CAD build for the part. Positions are in the model's coordinates, mm. A direction names the side the tool comes from. Round coordinates to 2 decimals unless told otherwise and drop trailing zeros. Loops run counter-clockwise (first coordinate to the right, second up) from the corner with the lowest first, then second, coordinate; pieces in that order, holes last. Notation, with made-up numbers: (-29.75, 38) - (-13.75, 38) arc R24 cw to (-13.75, 59) - close; hole circle Ø11 at (37.25, -28.75). An arc over 180 degrees is marked (long way). Use one line per item in the form item = value.
Solid Edge part; units mm, degrees
sketch "Sketch1" plane through (0, 0, 0) normal (0, -1, 0) x (1, 0, 0)
  line L0 (0, 0) -> (0, 40)
  line L1 (0, 40) -> (4, 40)
  line L2 (4, 40) -> (4, 4)
  line L3 (4, 4) -> (100, 4)
  line L4 (100, 4) -> (100, 0)
  line L5 (100, 0) -> (0, 0)
  dimension "D1" = 100
  dimension "D2" = 100
extrude "Protrusion1" add sketch "Sketch1" along normal mid plane 16
hole "Hole1" at (0, 0, 14) direction (1, 0, 0) diameter 2.459 end up to next
hole "Hole2" at (0, 0, 34) direction (1, 0, 0) diameter 2.459 end up to next
hole "Bohrung_3" at (14.002, 0, 0) direction (0, 0, 1) diameter 2.459 end up to next
hole "Hole3" at (90, 0, 0) direction (0, 0, 1) diameter 2.459 end up to next
properties material "Aluminiumlegierung:3.3535 , AlMg3, EN-AW 5754"
1) Two-plate mould, pull along Z, no slides. Class faces 1 (the flat face through (51, 0, 4)), 2 (the flat face through (100, 0, 2)), 3 (the cylindrical face through (1.972, 0.369, 15.173)): +Z half, -Z half, draft (parallel to the pull), parting line (faces both ways), or undercut.
Report:
face_1 = +Z half
face_2 = draft
face_3 = undercut
2) Slice it at A-A (x = 90). Write the cut outline in (y, z), plus the area to 3 significant figures.
Report:
outline = (-8, 0) - (-1.23, 0) - (-1.23, 4) - (-8, 4) - close; (1.23, 0) - (8, 0) - (8, 4) - (1.23, 4) - close
area = 54.2 mm^2
3) Slice it at D-D (x = 74.5). Write the cut outline in (y, z).
Report:
outline = (-8, 0) - (8, 0) - (8, 4) - (-8, 4) - close
4) Slice it at B-B (y = 0). Write the cut outline in (x, z), plus the area to 3 significant figures.
Report:
outline = (0, 0) - (12.77, 0) - (12.77, 4) - (4, 4) - (4, 12.77) - (0, 12.77) - close; (0, 15.23) - (4, 15.23) - (4, 32.77) - (0, 32.77) - close; (0, 35.23) - (4, 35.23) - (4, 40) - (0, 40) - close; (15.23, 0) - (88.77, 0) - (88.77, 4) - (15.23, 4) - close; (91.23, 0) - (100, 0) - (100, 4) - (91.23, 4) - close
area = 505 mm^2
5) Tool access for faces 4 (the cylindrical face through (1.97, 0.05, 32.77)), 5 (the flat face through (4, 0, 22)): list every direction of +Z, -Z, +X, -X, +Y, -Y with a clear straight run to the whole face (end or side of a thin tool).
Report:
face_4 = +X, -X
face_5 = +Z, +X, +Y, -Y
6) Slice it at C-C (z = 34). Write the cut outline in (x, y), plus the area to 3 significant figures.
Report:
outline = (0, -8) - (4, -8) - (4, -1.23) - (0, -1.23) - close; (0, 1.23) - (4, 1.23) - (4, 8) - (0, 8) - close
area = 54.2 mm^2
7) Drill centre lines: probe 1 along Z at (x, y) = (2.45, 0); probe 2 along X at (y, z) = (0, 0.9); probe 3 along Y at (x, z) = (90, 2.2). Where is each one in solid material? Low to high.
Report:
probe_1 = 0 to 12.77, 15.23 to 32.77, 35.23 to 40
probe_2 = 0 to 12.77, 15.23 to 88.77, 91.23 to 100
probe_3 = -8 to -1.23, 1.23 to 8
8) Flat gauge pins, fed straight in: pin 1 (8 mm diameter, centred on x = 38.5, y = 2.5, fed in from +Z); pin 2 (1.5 mm diameter, centred on y = -1, z = 25.5, fed in from +X). Where does each tip first touch, or does it go through?
Report:
pin_1 = 4
pin_2 = 4
